The figure shows three views and two pictorial views of one solid part (mm, origin at its lowest corner). Answer the questions. Round coordinates to 2 decimals unless told otherwise and drop trailing zeros. Write each loop counter-clockwise with the first axis right and the second up, starting at its lowest first coordinate (ties: lowest second). Pieces come first, ordered by that corner, then holes.
Item 1: Find the intervals of material crossed by probe 1 along Z at (x, y) = (2.95, 146); probe 2 along Z at (x, y) = (1.2, 24.13); probe 3 along Y at (x, z) = (2.1, 17.5), in increasing order.
Item 2: Each of these flat-tipped pins is pushed along its axis until it touches: pin 1 (1.6 mm diameter, centred on x = 1, y = 48.5, fed in from +Z); pin 2 (1 mm diameter, centred on x = 1, z = 19, fed in from -Y). Where does it stop, or does it pass through?
Item 3: Find section B-B on z = 35. Give the vertices of the cut face in (x, y) (1 decimal).
Item 4: Find section A-A on y = 141. Give the vertices of the cut face in (x, z) (1 decimal).
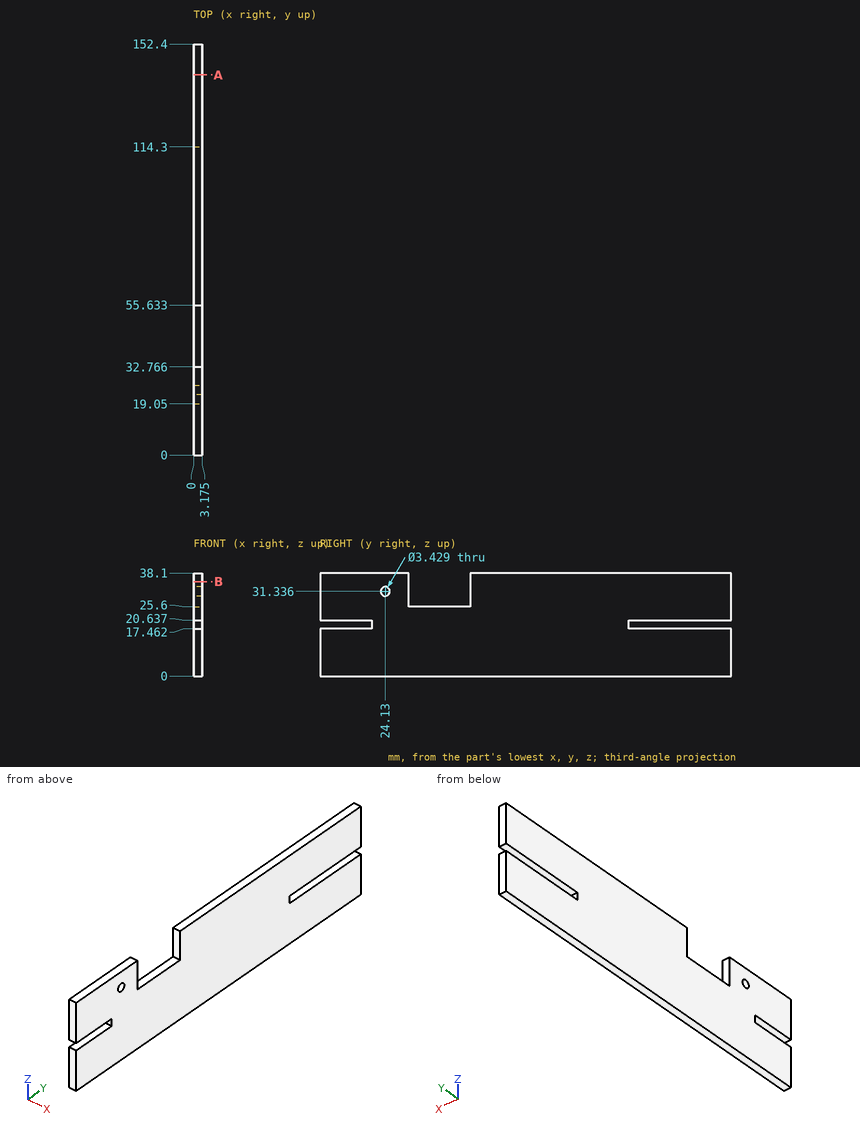
Check values:
1. probe 1: z = 0 to 17.46, 20.64 to 38.1
1. probe 2: z = 0 to 29.62, 33.05 to 38.1
1. probe 3: y = 19.05 to 114.3
2. pin 1: stops at z = 25.6
2. pin 2: stops at y = 19.05
3. outline: (0, 0) - (3.2, 0) - (3.2, 32.8) - (0, 32.8) - close; (0, 55.6) - (3.2, 55.6) - (3.2, 152.4) - (0, 152.4) - close
4. outline: (0, 0) - (3.2, 0) - (3.2, 17.5) - (0, 17.5) - close; (0, 20.6) - (3.2, 20.6) - (3.2, 38.1) - (0, 38.1) - close
